```python
from build123d import *

# Parameters (mm, degrees)
DODANIE_WYCI_GNI_CIE1_DEPTH = 46.5
WYTNIJ_WYCI_GNI_CIE1_DEPTH  = 2
SZKIC3_R                    = 3.25
WYTNIJ_WYCI_GNI_CIE2_DEPTH  = 2
DODANIE_WYCI_GNI_CIE2_DEPTH = 2
SZKIC5_W                    = 6.61
SZKIC5_H                    = 14.6
SZKIC5_W_2                  = 13.12
SZKIC5_H_2                  = 17.13
WYTNIJ_WYCI_GNI_CIE3_DEPTH  = 2


with BuildPart() as part:
    # Szkic1 → Dodanie-wyci_gni_cie1 (new body)
    with BuildSketch(Plane.XY):
        with BuildLine():
            Line((-51.3, -64), (51.3, -64))
            ThreePointArc((51.3, -64), (59.785281374, -60.485281374), (63.3, -52))
            Line((63.3, -52), (63.3, 52))
            ThreePointArc((63.3, 52), (59.785281374, 60.485281374), (51.3, 64))
            Line((51.3, 64), (-51.3, 64))
            ThreePointArc((-51.3, 64), (-59.785281374, 60.485281374), (-63.3, 52))
            Line((-63.3, 52), (-63.3, -52))
            ThreePointArc((-63.3, -52), (-59.785281374, -60.485281374), (-51.3, -64))
        make_face()
    extrude(amount=DODANIE_WYCI_GNI_CIE1_DEPTH)

    # Szkic2 → Wytnij-wyci_gni_cie1 (cut)
    with BuildSketch(Plane(origin=(0, 64, 0), x_dir=(1, 0, 0), z_dir=(0, 1, 0))):
        with BuildLine():
            Line((-48.65, -31.2), (-48.65, -40.2))
            ThreePointArc((-48.65, -40.2), (-48.210660172, -41.260660172), (-47.15, -41.7))
            Line((-47.15, -41.7), (46.85, -41.7))
            ThreePointArc((46.85, -41.7), (47.910660172, -41.260660172), (48.35, -40.2))
            Line((48.35, -40.2), (48.35, -31.2))
            ThreePointArc((48.35, -31.2), (47.910660172, -30.139339828), (46.85, -29.7))
            Line((46.85, -29.7), (-47.15, -29.7))
            ThreePointArc((-47.15, -29.7), (-48.210660172, -30.139339828), (-48.65, -31.2))
        make_face()
    wytnij_wyci_gni_cie1 = extrude(amount=-WYTNIJ_WYCI_GNI_CIE1_DEPTH, mode=Mode.SUBTRACT)

    # Szkic3 → Wytnij-wyci_gni_cie2 (cut)
    with BuildSketch(Plane.ZY.offset(63.3)):
        with BuildLine():
            ThreePointArc((29.5, -45.8), (28.439339828, -45.360660172), (28, -44.3))
            Line((28, -44.3), (28, 43.7))
            ThreePointArc((28, 43.7), (28.439339828, 44.760660172), (29.5, 45.2))
            Line((29.5, 45.2), (38.5, 45.2))
            ThreePointArc((38.5, 45.2), (39.560660172, 44.760660172), (40, 43.7))
            Line((40, 43.7), (40, -44.3))
            ThreePointArc((40, -44.3), (39.560660172, -45.360660172), (38.5, -45.8))
            Line((38.5, -45.8), (29.5, -45.8))
        make_face()
        with BuildLine():
            Line((13.72769909, -23), (13.72769909, -28.8))
            ThreePointArc((13.72769909, -28.8), (15.37769909, -30.45), (17.02769909, -28.8))
            Line((17.02769909, -28.8), (17.02769909, -23))
            ThreePointArc((17.02769909, -23), (15.37769909, -21.35), (13.72769909, -23))
        make_face()
        with BuildLine():
            Line((13.72769909, -3.9), (13.72769909, -9.7))
            ThreePointArc((13.72769909, -9.7), (15.37769909, -11.35), (17.02769909, -9.7))
            Line((17.02769909, -9.7), (17.02769909, -3.9))
            ThreePointArc((17.02769909, -3.9), (15.37769909, -2.25), (13.72769909, -3.9))
        make_face()
        with Locations((15.37769909, 10.1)):
            Circle(SZKIC3_R)
    extrude(amount=-WYTNIJ_WYCI_GNI_CIE2_DEPTH, mode=Mode.SUBTRACT)

    # Szkic3_3 → Dodanie-wyci_gni_cie2 (add)
    with BuildSketch(Plane.ZY.offset(63.3)):
        with BuildLine():
            Line((12.37769909, 31.6), (12.37769909, 23.1))
            ThreePointArc((12.37769909, 23.1), (12.670592309, 22.392893219), (13.37769909, 22.1))
            Line((13.37769909, 22.1), (17.37769909, 22.1))
            ThreePointArc((17.37769909, 22.1), (18.084805871, 22.392893219), (18.37769909, 23.1))
            Line((18.37769909, 23.1), (18.37769909, 31.6))
            ThreePointArc((18.37769909, 31.6), (18.084805871, 32.307106781), (17.37769909, 32.6))
            Line((17.37769909, 32.6), (13.37769909, 32.6))
            ThreePointArc((13.37769909, 32.6), (12.670592309, 32.307106781), (12.37769909, 31.6))
        make_face()
    extrude(amount=DODANIE_WYCI_GNI_CIE2_DEPTH)

    # Lustro1: Wytnij-wyci_gni_cie1 across plane
    add(wytnij_wyci_gni_cie1.mirror(Plane.ZX), mode=Mode.SUBTRACT)

    # Szkic5 → Wytnij-wyci_gni_cie3 (cut)
    with BuildSketch(Plane(origin=(63.3, 0, 0), x_dir=(0, 0, -1), z_dir=(1, 0, 0))):
        with BuildLine():
            Line((-39.86, 49.36), (-32.58, 49.36))
            ThreePointArc((-32.58, 49.36), (-31.165786438, 48.774213562), (-30.58, 47.36))
            Line((-30.58, 47.36), (-30.58, -18.86))
            ThreePointArc((-30.58, -18.86), (-31.165786438, -20.274213562), (-32.58, -20.86))
            Line((-32.58, -20.86), (-39.86, -20.86))
            ThreePointArc((-39.86, -20.86), (-41.274213562, -20.274213562), (-41.86, -18.86))
            Line((-41.86, -18.86), (-41.86, 47.36))
            ThreePointArc((-41.86, 47.36), (-41.274213562, 48.774213562), (-39.86, 49.36))
        make_face()
        with BuildLine():
            Line((-21.12, -44.41), (-12.62, -44.41))
            ThreePointArc((-12.62, -44.41), (-11.912893219, -44.702893219), (-11.62, -45.41))
            Line((-11.62, -45.41), (-11.62, -48))
            ThreePointArc((-11.62, -48), (-11.912893219, -48.707106781), (-12.62, -49))
            Line((-12.62, -49), (-21.12, -49))
            ThreePointArc((-21.12, -49), (-21.827106781, -48.707106781), (-22.12, -48))
            Line((-22.12, -48), (-22.12, -45.41))
            ThreePointArc((-22.12, -45.41), (-21.827106781, -44.702893219), (-21.12, -44.41))
        make_face()
        with Locations((-8.705, -4.63)):
            Rectangle(SZKIC5_W, SZKIC5_H)
        with Locations((-15.36, -26.725)):
            Rectangle(SZKIC5_W_2, SZKIC5_H_2)
        with Locations((-17.905, -4.63)):
            Rectangle(SZKIC5_W, SZKIC5_H)
        Polygon((-20.57, 9.9), (-5.24, 9.9), (-5.24, 12.83), (-7.82, 15.06), (-17.99, 15.06), (-20.57, 12.83), align=None)
        Polygon((-7.82, 27.77), (-5.24, 25.54), (-5.24, 22.61), (-20.57, 22.61), (-20.57, 25.54), (-17.99, 27.77), align=None)
        with Locations((-17.905, 42.04)):
            Rectangle(SZKIC5_W, SZKIC5_H)
        with Locations((-8.705, 42.04)):
            Rectangle(SZKIC5_W, SZKIC5_H)
    extrude(amount=-WYTNIJ_WYCI_GNI_CIE3_DEPTH, mode=Mode.SUBTRACT)


solid = part.part
```
Build history of the part. All positions in model axes, mm. A direction names the side the tool comes from. Give positions to 0.01 mm unless a question says otherwise; leave off trailing zeros. Order: outer loops, then holes, each group sorted by start corner. A loop starts at its lowest first (then second) coordinate and runs counter-clockwise, first axis right, second up. Notation, with made-up numbers: M 29,60 L 73,60 A28 cw 73,93 Z; hole C 36,64.5 d7. An arc over 180 degrees is marked long. Return JSON: item names as keys, results as strings.
Q1. Two-plate mould, pull along Y, no slides. Class faces 4 (the face through (59.88, 60.39, 22.92)), 5 (the face through (61.3, 42, 9)), 6 (the face through (-1, -64, 18)), 7 (the face through (-65.3, 27, 15)): pulls with the +Y half, pulls with the -Y half, needs draft (parallel to the pull), parting line crosses it, or undercut.
Answer list:
{"face 4": "pulls with the +Y half", "face 5": "undercut", "face 6": "pulls with the -Y half", "face 7": "needs draft"}
Q2. Band-saw the part on A-A (y = 4.5). Give the cut face in (x, z).
Answer list:
{"outline": "M -63.3,0 L 63.3,0 L 63.3,30.58 L 61.3,30.58 L 61.3,41.86 L 63.3,41.86 L 63.3,46.5 L -63.3,46.5 L -63.3,40 L -61.3,40 L -61.3,28 L -63.3,28 Z"}
Q3. Flat gauge pins, fed straight in: pin 1 (0.6 mm diameter, centred on x = 62, z = 18.5, fed in from +Y); pin 2 (4 mm diameter, centred on y = 12.5, z = 11.5, fed in from +X); pin 3 (2 mm diameter, centred on x = 62.5, z = 13, fed in from +Y). Where does each tip first touch, or does it go through?
Answer list:
{"pin 1": "stops at y = 57.99", "pin 2": "stops at x = 61.3", "pin 3": "stops at y = 58.32"}
Q4. Wall check: probe 1 along Z at (x, y) = (-62, 10); probe 2 along X at (y, z) = (-51, 18); probe 3 along X at (y, z) = (11.5, 15). Give the ranges that are in metal, low to high. Write a range as from..to.
Answer list:
{"probe 1": "z = 0..12.13, 18.63..28, 40..46.5", "probe 2": "x = -63.3..63.3", "probe 3": "x = -61.3..61.3"}
Q5. 3-axis set-ups, long thin cutter, end or side, ignore diameter. For faces 1 (the face through (-1, 62, 36)), 2 (the face through (61.3, -5, 18)), 3 (the face through (-61.3, 10, 15)): which of +Z, -Z, +X, -X, +Y, -Y reach the whole face in a straight line?
Answer list:
{"face 1": "+Y", "face 2": "+X", "face 3": "-X"}
